CAD build for the part. Positions are in the model's coordinates, mm. Face numbers are marked on the shaded views. A direction names the side the tool comes from. Give positions to 0.01 mm unless a question says otherwise; leave off trailing zeros. Loops run counter-clockwise (first coordinate to the right, second up) from the corner with the lowest first, then second, coordinate; pieces in that order, holes last.
Autodesk Inventor part; units mm, degrees
ref_plane "YZ Plane" through (0, 0, 0) normal (1, 0, 0) x (0, 1, 0)
ref_plane "XZ Plane" through (0, 0, 0) normal (0, 1, 0) x (-1, 0, 0)
ref_plane "XY Plane" through (0, 0, 0) normal (0, 0, 1) x (1, 0, 0)
sketch "スケッチ1" plane through (0, 0, 0) normal (0, 0, 1) x (1, 0, 0)
  arc A0 (-5.1, 0) -> (5.1, 0) centre (0, 0) ccw
  line L0 (-15, 8) -> (15, 8)
  line L1 (15, 8) -> (15, 0)
  line L2 (15, 0) -> (5.1, 0)
  line L3 (-15, 0) -> (-15, 8)
  arc A1 (5.1, 0) -> (-5.1, 0) centre (0, 0) ccw
  line L4 (5.1, 0) -> (-5.1, 0)
  line L5 (-5.1, 0) -> (-15, 0)
  dimension "d0" = 10.2
  dimension "d1" = 30
  dimension "d2" = 15
  dimension "d3" = 8
  dimension "d4" = 0
extrude "押し出し1" add sketch "スケッチ1" along normal blind 30 contours L5 L3 L0 L1 L2 A1
sketch "スケッチ2" plane through (-15, 0, 0) normal (0, -1, 0) x (1, 0, 0)
  line L0 (9.9, 30) -> (0, 30)
  line L1 (0, 0) -> (9.9, 0)
  line L2 (0, 30) -> (4.95, 30)
  line L3 (4.95, 30) -> (4.95, 0)
  line L4 (4.95, 0) -> (0, 0)
  line L5 (0, 0) -> (0, 30)
  line L6 (30, 30) -> (25.05, 30)
  line L7 (25.05, 30) -> (25.05, 0)
  line L8 (25.05, 0) -> (30, 0)
  line L9 (30, 0) -> (30, 30)
  point P0 (15, 0)
  dimension "d7" = 30
  dimension "d8" = 4.95
extrude "押し出し2" add sketch "スケッチ2" along normal blind 2
fillet "フィレット1" radius 1 4 edges at (-10.05, -2, 15) (-10.05, 0, 15) (10.05, 0, 15) (10.05, -2, 15)
sketch "スケッチ3" plane through (-15, 8, 0) normal (0, 1, 0) x (1, 0, 0)
  line L0 (0, -30) -> (30, -30)
  line L1 (30, 0) -> (30, -30)
  line L2 (30, 0) -> (0, 0)
  line L3 (0, 0) -> (0, -30)
  point P0 (15, 0)
  point P1 (5, -5)
  point P2 (5, -25)
  point P3 (25, -25)
  point P4 (25, -5)
  dimension "d11" = 5
  dimension "d12" = 5
  dimension "d13" = 5
  dimension "d14" = 5
  dimension "d15" = 5
  dimension "d16" = 5
  dimension "d17" = 5
  dimension "d18" = 5
hole "Hole2" at (-10, 8, 5) at (-10, 8, 25) at (10, 8, 25) at (10, 8, 5) direction (0, -1, 0) diameter 3 end through all
properties part number "poleHolderA"
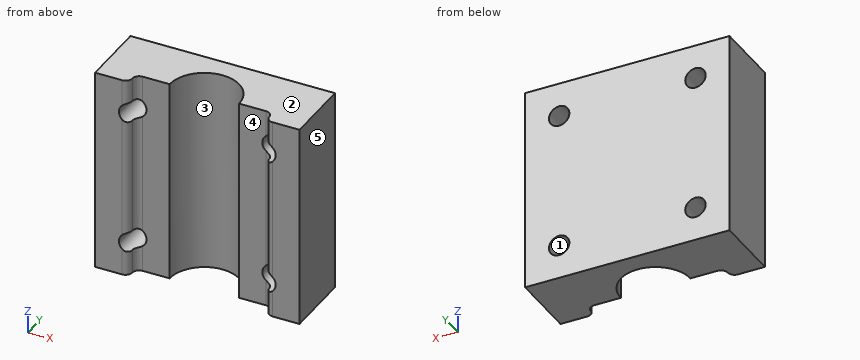
1. Tool access for the marked faces 4 and 5: list every direction of +Z, -Z, +X, -X, +Y, -Y with a clear straight run to the whole face (end or side of a thin tool).
Responses:
face 4: +Z, -Z, -Y
face 5: +Z, -Z, +X, +Y, -Y
2. Pull direction Z, two halves, no side cores. Call the marked faces 1, 2 and 3: released by +Z, released by -Z, zero draft, split by the parting line, or undercut.
Responses:
face 1: undercut
face 2: released by +Z
face 3: zero draft
3. Saw through at B-B, the plane y = 2. List the corners of the cut face in (x, z), and give its area (3 significant figures).
Responses:
outline: (-15, 0) - (-4.69, 0) - (-4.69, 30) - (-15, 30) - close; (4.69, 0) - (15, 0) - (15, 30) - (4.69, 30) - close; hole circle Ø3 at (-10, 5); hole circle Ø3 at (-10, 25); hole circle Ø3 at (10, 5); hole circle Ø3 at (10, 25)
area: 590 mm2
4. Drop flat-ended pins along their axis: pin 1 (1.8 mm diameter, centred on x = 10, z = 25, fed in from +Y); pin 2 (1.2 mm diameter, centred on x = 6.5, z = 15, fed in from -Y). Give the stop position or say it passes through.
Responses:
pin 1: passes through
pin 2: stops at y = 0
5. Saw through at A-A, the plane z = 25. List the corners of the cut face in (x, y).
Responses:
outline: (-15, -2) - (-11.5, -2) - (-11.5, 8) - (-15, 8) - close; (-8.5, 0) - (-5.1, 0) arc R5.1 cw to (5.1, 0) - (8.5, 0) - (8.5, 8) - (-8.5, 8) - close; (11.5, -2) - (15, -2) - (15, 8) - (11.5, 8) - close
6. Saw through at D-D, the plane x = 0. List the corners of the cut face in (y, z), and give its area (3 significant figures).
Responses:
outline: (5.1, 0) - (8, 0) - (8, 30) - (5.1, 30) - close
area: 87.0 mm2
7. Probe line 1 along X through (y, z) = (0.25, 5); line 2 along Z through (x, y) = (-10, 4.25); line 3 along X through (y, z) = (6, 5). List the from-to ranges inside material, lowest first.
Responses:
line 1: x = -15 to -11.5, -8.5 to -5.09, 5.09 to 8.5, 11.5 to 15
line 2: z = 0 to 3.5, 6.5 to 23.5, 26.5 to 30
line 3: x = -15 to -11.5, -8.5 to 8.5, 11.5 to 15
